Read the model definition and answer for the solid it produces. Units are mm, in the model's axes. Face numbers are marked on the shaded views. A direction names the side the tool comes from. Round coordinates to 2 decimals unless told otherwise and drop trailing zeros. Order: outer loops, then holes, each group sorted by start corner. A loop starts at its lowest first (then second) coordinate and runs counter-clockwise, first axis right, second up. Notation, with made-up numbers: M -35.5,-25 L -0.5,-25 A17 cw -0.5,-6 Z; hole C -25,29.25 d1. An arc over 180 degrees is marked long. Use one line per item in the form item = value. Start each with the question number.
from build123d import *

# Parameters (mm, degrees)
PAD013_DEPTH            = 2
SKETCH020_R             = 4
PAD014_DEPTH            = 3.5
HOLE_D                  = 3.4
HOLE_DEPTH              = 25
HOLE_CSINK_D            = 6.7
HOLE_CSINK_ANGLE        = 90
BODY004_PLACEMENT_ANGLE = 180


with BuildPart() as part:
    # Sketch019 → Pad013 (new body)
    with BuildSketch(Plane.XY):
        with BuildLine():
            Line((-32.3, -39.278), (-32.3, 39.278))
            ThreePointArc((-28.3, 43.278), (-31.128427, 42.106427), (-32.3, 39.278))
            Line((-28.3, 43.278), (28.3, 43.278))
            ThreePointArc((32.3, 39.278), (31.128427, 42.106427), (28.3, 43.278))
            Line((32.3, 39.278), (32.3, -39.278))
            ThreePointArc((28.3, -43.278), (31.128427, -42.106427), (32.3, -39.278))
            Line((28.3, -43.278), (-28.3, -43.278))
            ThreePointArc((-32.3, -39.278), (-31.128427, -42.106427), (-28.3, -43.278))
        make_face()
    extrude(amount=PAD013_DEPTH)

    # Sketch020 → Pad014 (join)
    with BuildSketch(Plane.XY):
        with Locations((-26.5, 37.478)):
            Circle(SKETCH020_R)
        with Locations((26.5, 37.478)):
            Circle(SKETCH020_R)
        with Locations((26.5, 20.522)):
            Circle(SKETCH020_R)
        with Locations((26.5, -37.478)):
            Circle(SKETCH020_R)
        with Locations((-26.5, -37.478)):
            Circle(SKETCH020_R)
        with Locations((-26.5, 20.522)):
            Circle(SKETCH020_R)
    extrude(amount=PAD014_DEPTH)

    # Hole
    with Locations(Plane(origin=(0, 0, 0), x_dir=(1, 0, 0), z_dir=(0, 0, -1))):
        with Locations((-26.5, -37.478), (26.5, -37.478), (26.5, -20.522), (26.5, 37.478), (-26.5, 37.478), (-26.5, -20.522)):
            CounterSinkHole(HOLE_D / 2, HOLE_CSINK_D / 2, depth=HOLE_DEPTH, counter_sink_angle=HOLE_CSINK_ANGLE)


with BuildPart() as part_1:
    # Body004 placement: moved
    add(part.part.moved(Location((0, 0, 61))).rotate(Axis((0, 0, 61), (0, 1, 0)), BODY004_PLACEMENT_ANGLE))


solid = part_1.part
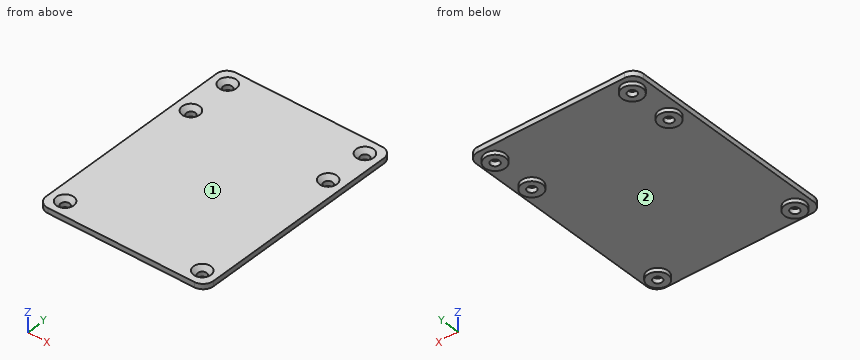
Item 1: Section C-C (y = 30.5) is taken. Write down the section's boundary in (x, z), and give its area (3 significant figures).
Item 2: Given P1, Ø3, axis at x = 26.5, y = 20.522, coming from the +Z side; P2, Ø19.5, axis at x = -12, y = -5, coming from the -Z side; P3, Ø5.5, axis at x = 26.5, y = -37.478, coming from the +Z side; P4, Ø4, axis at x = -26.5, y = 20.522, coming from the +Z side, each flat-ended and moving along its own axis, determine where each tip first touches the part or whether it passes through.
Item 3: Section D-D (x = 12) is taken. Write down the section's boundary in (y, z), and give its area (3 significant figures).
Item 4: Section A-A (z = 58.1) is taken. Give the number of separate pieces and of enclosed holes in the cut face, and give its area (3 significant figures).
Item 5: A tool of negligible diameter and unlimited length cuts with its end or side. For the marked faces 1 and 2, from which of +Z, -Z, +X, -X, +Y, -Y can it reach the whole face along a straight path? Write none if from no direction.
Item 6: Find the intervals of material crossed by L1, parallel to Y at x = -26.5, z = 57.9; L2, parallel to X at y = 37, z = 59.8; L3, parallel to X at y = 19, z = 60.3, in increasing order. Write a range as [from, to].
The answers:
q1.outline = M -32.3,59 L 32.3,59 L 32.3,61 L -32.3,61 Z
q1.area = 129 mm²
q2.P1 = through
q2.P2 = 59
q2.P3 = 60.4
q2.P4 = 59.65
q3.outline = M -43.28,59 L 43.28,59 L 43.28,61 L -43.28,61 Z
q3.area = 173 mm²
q4.separate_pieces = 6
q4.enclosed_holes = 6
q4.area = 247 mm²
q5.face_1 = +Z, +X, -X, +Y, -Y
q5.face_2 = -Z
q6.L1 = [-41.48, -39.18], [-35.78, -33.48], [16.52, 18.82], [22.22, 24.52], [33.48, 35.78], [39.18, 41.48]
q6.L2 = [-32.3, -28.6], [-24.4, 24.4], [28.6, 32.3]
q6.L3 = [-32.3, -28.67], [-24.33, 24.33], [28.67, 32.3]
